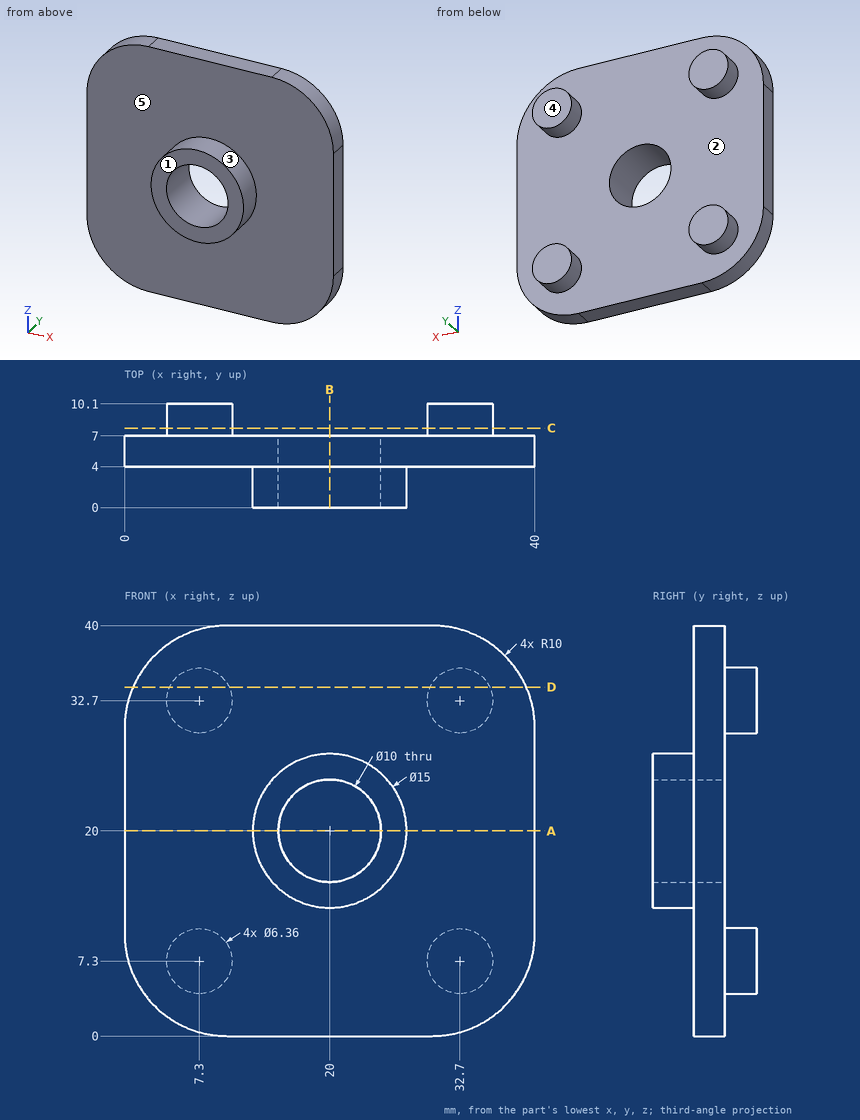
For this review, use the dimensioned drawing (mm, ordinates from the lowest corner) and the shaded views. A direction names the side the tool comes from. Coordinates: 2 decimals unless noted, no trailing zeros. Loops run counter-clockwise (first coordinate to the right, second up) from the corner with the lowest first, then second, coordinate; pieces in that order, holes last. Notation, with made-up numbers: (11, -2.75) - (37, -2.75) arc R20 cw to (37, 14.25) - close; hole circle Ø2 at (30, 85.25). An arc over 180 degrees is marked (long way). Use one line per item in the form item = value. Start each with the question number.
1) Take a section at C-C (y = 7.75). State the section outline as (x, z) points.
2) For the marked faces 4 and 5, list the 3-axis set-ups (+Z, -Z, +X, -X, +Y, -Y) from which the entire face can be reached by the end or side of a thin tool; tool diameter is ignored.
3) Take a section at A-A (z = 20). State the section outline as (x, y) points, plus the area to 3 significant figures.
4) To check wall thickness, follow probe 1 along X at (y, z) = (4.25, 20); probe 2 along Z at (x, y) = (20, 3.5). State the ranges of each line that lie inside material, in increasing order. Write a range as from..to.
5) For pin 1 (20 mm diameter, centred on x = 14.5, z = 18.5, fed in from +Y); pin 2 (6 mm diameter, centred on x = 20, z = 20, fed in from -Y); pin 3 (1 mm diameter, centred on y = 4, z = 7.5, fed in from +X); pin 4 (5 mm diameter, centred on x = 9.5, z = 10, fed in from -Y), all flat-tipped, find the tip position at first contact; note any pin that passes through.
6) Take a section at D-D (z = 34). State the section outline as (x, y) points, plus the area to 3 significant figures.
7) Draft analysis for pull direction Z (two halves, no side actions). For the marked faces 1, 2 and 3, state which applies: released by +Z, released by -Z, zero draft, split by the parting line, or undercut.
8) Take a section at B-B (x = 20). State the section outline as (y, z) points, plus the area to 3 significant figures.
From the geometry:
q1.outline = circle Ø6.36 at (7.3, 7.3); circle Ø6.36 at (7.3, 32.7); circle Ø6.36 at (32.7, 7.3); circle Ø6.36 at (32.7, 32.7)
q2.face_4 = +Z, -Z, +X, -X, +Y
q2.face_5 = -Y
q3.outline = (0, 4) - (12.5, 4) - (12.5, 0) - (15, 0) - (15, 7) - (0, 7) - close; (25, 0) - (27.5, 0) - (27.5, 4) - (40, 4) - (40, 7) - (25, 7) - close
q3.area = 110 mm2
q4.probe_1 = 0..15, 25..40
q4.probe_2 = 12.5..15, 25..27.5
q5.pin_1 = 7
q5.pin_2 = through
q5.pin_3 = 39.8
q5.pin_4 = 4
q6.outline = (0.83, 4) - (39.17, 4) - (39.17, 7) - (35.6, 7) - (35.6, 10.1) - (29.8, 10.1) - (29.8, 7) - (10.2, 7) - (10.2, 10.1) - (4.4, 10.1) - (4.4, 7) - (0.83, 7) - close
q6.area = 151 mm2
q7.face_1 = zero draft
q7.face_2 = undercut
q7.face_3 = split by the parting line
q8.outline = (0, 12.5) - (4, 12.5) - (4, 0) - (7, 0) - (7, 15) - (0, 15) - close; (0, 25) - (7, 25) - (7, 40) - (4, 40) - (4, 27.5) - (0, 27.5) - close
q8.area = 110 mm2
